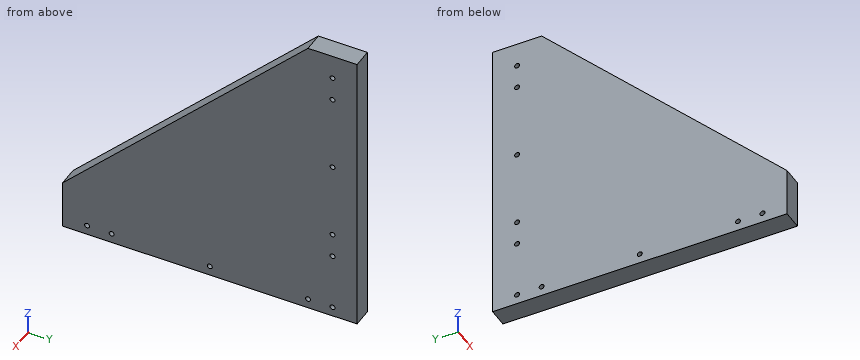
from build123d import *

# Parameters (mm, degrees)
F1_DEPTH = 40
F4_D     = 10


with BuildPart() as f1:
    # F0 (on Right) → F1 (new body)
    with BuildSketch(Plane.YZ):
        Polygon((-600, 0), (0, 0), (0, 600), (-100, 600), (-600, 100), align=None)
    extrude(amount=F1_DEPTH)

    # F4 (through all)
    with Locations(Plane(origin=(0, 0, 0), x_dir=(0, -1, 0), z_dir=(-1, 0, 0))):
        with Locations((50, 20), (100, 20), (300, 20), (500, 20), (550, 20), (50, 138), (50, 188), (50, 344), (50, 500), (50, 550)):
            Hole(F4_D / 2)


solid = f1.part
Read the model definition and answer for the solid it produces. Units are mm, in the model's axes. Give positions to 0.01 mm unless a question says otherwise; leave off trailing zeros. Loops run counter-clockwise (first coordinate to the right, second up) from the corner with the lowest first, then second, coordinate; pieces in that order, holes last. Notation, with made-up numbers: (42.25, 78.5) - (70.25, 78.5) arc R23 cw to (70.25, 98.5) - close; hole circle Ø5 at (87.25, 19.25). An arc over 180 degrees is marked (long way). Answer as CSV lines item,"result". Start each with the question number.
1) Find section B-B (z = 109). Write down the section's boundary in (x, y), then the cut area to 3 significant figures.
2) Find section A-A (x = 14). State how many separate pieces and enclosed holes the cut face has, then the cut area to 3 significant figures.
3) Find section C-C (y = -466.5). Write down the section's boundary in (x, z), then the cut area to 3 significant figures.
4) Straight lines are drawn through the part: L1, parallel to Y at x = 15.5, z = 344; L2, parallel to Y at x = 12, z = 500; L3, parallel to Z at x = 13, y = -104. For each, find the intervals that lie inside material, in ascending order. Write a range as from..to.
5) Each of these flat-tipped pins is pushed along its axis until it touches: pin 1 Ø1 at (x, y) = (23.5, -400) entering from +Z; pin 2 Ø9 at (y, z) = (-50, 500) entering from -X; pin 3 Ø4 at (x, y) = (24, -385.5) entering from +Z; pin 4 Ø1 at (x, y) = (4.5, -341) entering from +Z. Where does it stop, or does it pass through?
Findings below:
1,outline,"(0, -591) - (40, -591) - (40, 0) - (0, 0) - close"
1,area,"23,600 mm^2"
2,separate pieces,"1"
2,enclosed holes,"10"
2,area,"234,000 mm^2"
3,outline,"(0, 0) - (40, 0) - (40, 233.5) - (0, 233.5) - close"
3,area,"9,340 mm^2"
4,L1,"-356..-55, -45..0"
4,L2,"-200..-55, -45..0"
4,L3,"0..17, 23..596"
5,pin 1,"z = 300.5"
5,pin 2,"through"
5,pin 3,"z = 316.5"
5,pin 4,"z = 359.5"
